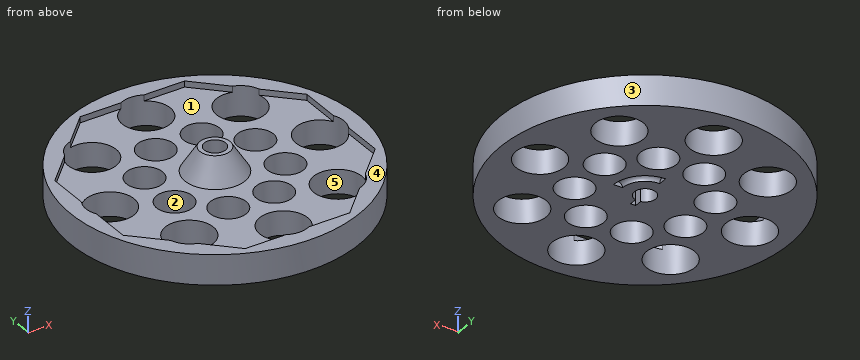
```python
from build123d import *

# Parameters (mm, degrees)
SKETCH_R       = 48
SKETCH_R_2     = 8
SKETCH_R_3     = 6
PAD_DEPTH      = 10
POCKET_DEPTH   = 2
CYLINDER_R     = 3.55
CYLINDER_DEPTH = 16
BOX_W          = 3
BOX_H          = 1.7
BOX_DEPTH      = 9.5
TORUS_R        = 1.5
TORUS_ANGLE    = 90


with BuildPart() as part:
    # Sketch → Pad (new body)
    with BuildSketch(Plane.XY):
        Circle(SKETCH_R)
        with Locations((0, 35)):
            Circle(SKETCH_R_2, mode=Mode.SUBTRACT)
        with Locations((24.748737, 24.748737)):
            Circle(SKETCH_R_2, mode=Mode.SUBTRACT)
        with Locations((35, 0)):
            Circle(SKETCH_R_2, mode=Mode.SUBTRACT)
        with Locations((24.748737, -24.748737)):
            Circle(SKETCH_R_2, mode=Mode.SUBTRACT)
        with Locations((0, -35)):
            Circle(SKETCH_R_2, mode=Mode.SUBTRACT)
        with Locations((-24.748737, -24.748737)):
            Circle(SKETCH_R_2, mode=Mode.SUBTRACT)
        with Locations((-35, 0)):
            Circle(SKETCH_R_2, mode=Mode.SUBTRACT)
        with Locations((-24.748737, 24.748737)):
            Circle(SKETCH_R_2, mode=Mode.SUBTRACT)
        with Locations((-7.653669, -18.477591)):
            Circle(SKETCH_R_3, mode=Mode.SUBTRACT)
        with Locations((7.653669, -18.477591)):
            Circle(SKETCH_R_3, mode=Mode.SUBTRACT)
        with Locations((18.477591, -7.653669)):
            Circle(SKETCH_R_3, mode=Mode.SUBTRACT)
        with Locations((18.477591, 7.653669)):
            Circle(SKETCH_R_3, mode=Mode.SUBTRACT)
        with Locations((7.653669, 18.477591)):
            Circle(SKETCH_R_3, mode=Mode.SUBTRACT)
        with Locations((-7.653669, 18.477591)):
            Circle(SKETCH_R_3, mode=Mode.SUBTRACT)
        with Locations((-18.477591, 7.653669)):
            Circle(SKETCH_R_3, mode=Mode.SUBTRACT)
        with Locations((-18.477591, -7.653669)):
            Circle(SKETCH_R_3, mode=Mode.SUBTRACT)
    extrude(amount=PAD_DEPTH)

    # Sketch001 (on Face19 of Pad) → Pocket (cut)
    with BuildSketch(Plane.XY.offset(10)):
        Polygon((42.036519, 17.412096), (17.412096, 42.036519), (-17.412096, 42.036519), (-42.036519, 17.412096), (-42.036519, -17.412096), (-17.412096, -42.036519), (17.412096, -42.036519), (42.036519, -17.412096), align=None)
    extrude(amount=-POCKET_DEPTH, mode=Mode.SUBTRACT)

    # Cone → Cone (revolve)
    with BuildSketch(Plane(origin=(0, 0, 8), x_dir=(1, 0, 0), z_dir=(0, -1, 0))):
        Polygon((0, 0), (10, 0), (5, 8), (0, 8), align=None)
    revolve(axis=Axis((0, 0, 8), (0, 0, 1)))

    # Cylinder → Cylinder (cut)
    with BuildSketch(Plane(origin=(0, 0, 16), x_dir=(-1, 0, 0), z_dir=(0, 0, -1))):
        Circle(CYLINDER_R)
    extrude(amount=CYLINDER_DEPTH, mode=Mode.SUBTRACT)

    # Box → Box (cut)
    with BuildSketch(Plane(origin=(-0.8, -3, 0), x_dir=(0, -1, 0), z_dir=(0, 0, 1))):
        with Locations((1.5, 0.85)):
            Rectangle(BOX_W, BOX_H)
    extrude(amount=BOX_DEPTH, mode=Mode.SUBTRACT)

    # Torus → Torus (revolve, cut)
    with BuildSketch(Plane.XZ):
        with Locations((9, 0)):
            Circle(TORUS_R)
    revolve(axis=Axis((0, 0, 0), (0, 0, 1)), revolution_arc=TORUS_ANGLE, mode=Mode.SUBTRACT)


solid = part.part
```
Work out the finished part from the listing and answer in its coordinate system (mm). Face numbers are marked on the shaded views. A direction names the side the tool comes from. Round coordinates to 2 decimals unless told otherwise and drop trailing zeros. Write each loop counter-clockwise with the first axis right and the second up, starting at its lowest first coordinate (ties: lowest second). Pieces come first, ordered by that corner, then holes. Notation, with made-up numbers: (75, 41.25) - (129, 41.25) arc R24 ccw to (129, 68.25) - close; hole circle Ø11 at (76, 18). An arc over 180 degrees is marked (long way). Return JSON: item names as keys, results as strings. Group by question number.
Q1. The mould has two halves that part along X. Classify the marked faces 3, 4 and 5: released by +X, released by -X, zero draft, split by the parting line, or undercut.
Q2. The part is cut by section C-C on z = 6.5. Count the separate pieces of the cut face and the enclosed holes in it, then the cut area to 3 significant figures.
Q3. For the marked faces 1 and 2, determine the directions among +Z, -Z, +X, -X, +Y, -Y from which every point of the face is accessible in a straight line to the end or side of a thin tool.
Q4. Each of these flat-tipped pins is pushed along its axis until it touches: pin 1 Ø6 at (y, z) = (-17.5, 10) entering from +X; pin 2 Ø3 at (x, z) = (28.5, 5.5) entering from +Y; pin 3 Ø1.2 at (y, z) = (8.5, 0.5) entering from +X; pin 4 Ø4 at (x, z) = (22.5, 13.5) entering from +Y. Where does it stop, or does it pass through?
Q5. Find the intervals of material crossed by L1, parallel to Y at x = 0, z = 6.75; L2, parallel to X at y = -29, z = 1; L3, parallel to Y at x = -6, z = 1, in increasing order.
Q6. The part is cut by section A-A on x = 35. Write down the section's boundary in (y, z).
Solved:
{
 "1": {"face 3": "split by the parting line", "face 4": "zero draft", "face 5": "undercut"},
 "2": {"separate pieces": "1", "enclosed holes": "17", "area": "4,680 mm²"},
 "3": {"face 1": "+Z", "face 2": "+Z, -Z"},
 "4": {"pin 1": "x = 45.76", "pin 2": "y = 39.69", "pin 3": "x = 47.35", "pin 4": "through"},
 "5": {"L1": "-48 to -43, -27 to -6, 3.55 to 27, 43 to 48", "L2": "-38.25 to -31.53, -17.97 to -5.29, 5.29 to 17.97, 31.53 to 38.25", "L3": "-47.62 to -40.29, -29.71 to -24.25, -12.71 to 12.71, 24.25 to 29.71, 40.29 to 47.62"},
 "6": {"outline": "(-32.85, 0) - (-8, 0) - (-8, 8) - (-24.45, 8) - (-24.45, 10) - (-32.85, 10) - close; (8, 0) - (32.85, 0) - (32.85, 10) - (24.45, 10) - (24.45, 8) - (8, 8) - close"}
}
